Here's the drawing with two shaded views (mm, measured from the low corner). I have some questions. A direction names the side the tool comes from. Coordinates: 2 decimals unless noted, no trailing zeros. Write each loop counter-clockwise with the first axis right and the second up, starting at its lowest first coordinate (ties: lowest second). Pieces come first, ordered by that corner, then holes. Notation, with made-up numbers: (70.5, 71.5) -> (122.5, 71.5) arc R7 ccw to (122.5, 76.5) -> close; hole circle Ø10 at (14, -8.75). An arc over 180 degrees is marked (long way). Put each result on its own line as item: value.
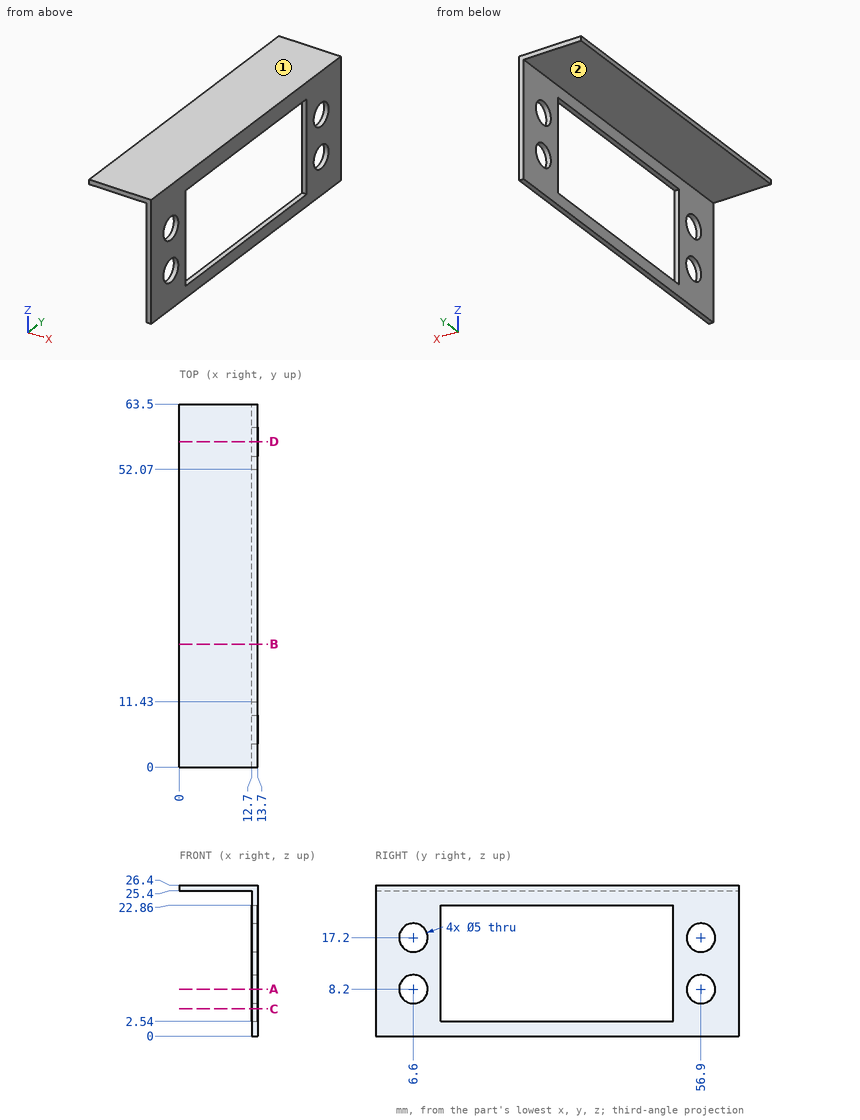
Item 1: Imagine slicing it at D-D on y = 56.9. Write out the boundary of the cut face in (x, z), then the cut area to 3 significant figures.
Output:
outline: (0, 25.4) -> (12.7, 25.4) -> (12.7, 19.7) -> (13.7, 19.7) -> (13.7, 26.4) -> (0, 26.4) -> close; (12.7, 0) -> (13.7, 0) -> (13.7, 5.7) -> (12.7, 5.7) -> close; (12.7, 10.7) -> (13.7, 10.7) -> (13.7, 14.7) -> (12.7, 14.7) -> close
area: 29.1 mm²
Item 2: Imagine slicing it at B-B on y = 21.5. Write out the boundary of the cut face in (x, z).
Output:
outline: (0, 25.4) -> (12.7, 25.4) -> (12.7, 22.86) -> (13.7, 22.86) -> (13.7, 26.4) -> (0, 26.4) -> close; (12.7, 0) -> (13.7, 0) -> (13.7, 2.54) -> (12.7, 2.54) -> close
Item 3: Imagine slicing it at A-A on z = 8.2. Write out the boundary of the cut face in (x, y).
Output:
outline: (12.7, 0) -> (13.7, 0) -> (13.7, 4.1) -> (12.7, 4.1) -> close; (12.7, 9.1) -> (13.7, 9.1) -> (13.7, 11.43) -> (12.7, 11.43) -> close; (12.7, 52.07) -> (13.7, 52.07) -> (13.7, 54.4) -> (12.7, 54.4) -> close; (12.7, 59.4) -> (13.7, 59.4) -> (13.7, 63.5) -> (12.7, 63.5) -> close
Item 4: Which directions (+Z, -Z, +X, -X, +Y, -Y) give clear straight access to the entire face, cutting with the end or side of a thin tool? Please do the marked faces 1 and 2.
Output:
face 1: +Z, +X, -X, +Y, -Y
face 2: -Z, -X, +Y, -Y
Item 5: Imagine slicing it at C-C on z = 4.75. Write out the boundary of the cut face in (x, y).
Output:
outline: (12.7, 0) -> (13.7, 0) -> (13.7, 11.43) -> (12.7, 11.43) -> close; (12.7, 52.07) -> (13.7, 52.07) -> (13.7, 63.5) -> (12.7, 63.5) -> close
Item 6: Please list where these lines run through material, in increasing order: line 1 along Y through (x, z) = (13.35, 17.2); line 2 along Z through (x, y) = (11.75, 27.5); line 3 along X through (y, z) = (28, 2). Write a range as from..to.
Output:
line 1: y = 0..4.1, 9.1..11.43, 52.07..54.4, 59.4..63.5
line 2: z = 25.4..26.4
line 3: x = 12.7..13.7
Item 7: For P1, Ø0.5, axis at x = 13.5, z = 14, coming from the -Y side; P2, Ø4, axis at x = 3.5, y = 21.5, coming from the -Z side; P3, Ø3, axis at y = 56.9, z = 8.2, coming from the -X side; P4, Ø8, axis at y = 6.6, z = 8.2, coming from the -X side, each with a flat end and sliding along its axis, tell me the tip position at first contact or that it passes through.
Output:
P1: stops at y = 0
P2: stops at z = 25.4
P3: passes through
P4: stops at x = 12.7
